Autodesk Inventor part; units mm, degrees
ref_plane "YZ Plane" through (0, 0, 0) normal (1, 0, 0) x (0, 1, 0)
ref_plane "XZ Plane" through (0, 0, 0) normal (0, 1, 0) x (-1, 0, 0)
ref_plane "XY Plane" through (0, 0, 0) normal (0, 0, 1) x (1, 0, 0)
sketch "Sketch1" plane through (0, 0, 0) normal (0, 1, 0) x (-1, 0, 0)
  line L0 (25, 25) -> (-25, 25)
  line L1 (-25, 25) -> (-25, -25)
  line L2 (-25, -25) -> (25, -25)
  line L3 (25, -25) -> (25, 25)
  point P0 (0, 0)
  dimension "d0" = 50
  dimension "d1" = 50
  dimension "d2" = 25
  dimension "d3" = 25
extrude "Extrusion1" add sketch "Sketch1" along normal blind 5
sketch "Sketch2" plane through (0, 0, 0) normal (0, -1, 0) x (1, 0, 0)
  circle A0 centre (0, 0) radius 8
  dimension "d6" = 16
extrude "Extrusion2" add sketch "Sketch2" along normal blind 10
sketch "Sketch3" plane through (0, 5, 0) normal (0, 1, 0) x (1, 0, 0)
  line L0 (0, -3) -> (0, -3)
  line L1 (3, 0) -> (3, 0)
  line L2 (0, 3) -> (0, 3)
  line L3 (-3, 0) -> (-3, 0)
  arc A0 (-3, 0) -> (0, -3) centre (0, 0) ccw
  arc A1 (0, 3) -> (-3, 0) centre (0, 0) ccw
  arc A2 (3, 0) -> (0, 3) centre (0, 0) ccw
  arc A3 (0, -3) -> (3, 0) centre (0, 0) ccw
  point P0 (0, 0)
  dimension "d9" = 6
  dimension "d10" = 6
  dimension "d11" = 3
  dimension "d12" = 3
  dimension "d19" = 3
extrude "Extrusion3" cut sketch "Sketch3" against normal blind 6
sketch "Sketch4" plane through (0, 5, 0) normal (0, 1, 0) x (1, 0, 0)
  line L0 (-5, -5) -> (-5, 5)
  line L1 (-25, 25) -> (-25, -25)
  circle A0 centre (-15, 0) radius 2.5
  line L2 (5, -5) -> (-5, -5)
  line L3 (-5, 5) -> (5, 5)
  circle A1 centre (15, 0) radius 2.5
  line L4 (25, -25) -> (25, 25)
  point P0 (0, 0)
  dimension "d15" = 5
  dimension "d20" = 10
  dimension "d21" = 10
extrude "Extrusion4" cut sketch "Sketch4" against normal blind 3
fillet "Fillet1" radius 5 4 edges at (25, 2.5, 25) (25, 2.5, -25) (-25, 2.5, -25) (-25, 2.5, 25)
sketch "Sketch5" plane through (0, 0, 0) normal (1, 0, 0) x (0, 1, 0)
  line L0 (0, 8) -> (-10, 8)
  line L1 (0, 8) -> (0, 8.5)
  line L2 (0, 20) -> (0, -20)
  line L3 (-10, 8) -> (-10, -8)
  line L4 (-10, 8) -> (0, 8)
  line L5 (-10, 0) -> (0, 0)
  arc A0 (0, 8.5) -> (-10, 8) centre (-2.7668, -36.4149) ccw
  dimension "d23" = 0.5
  dimension "d25" = 45
revolve "Revolution1" add sketch "Sketch5" angle 360 about axis through (0, -10, 0) along (0, 1, 0) contours L0 A0 L1
properties part number "Base"
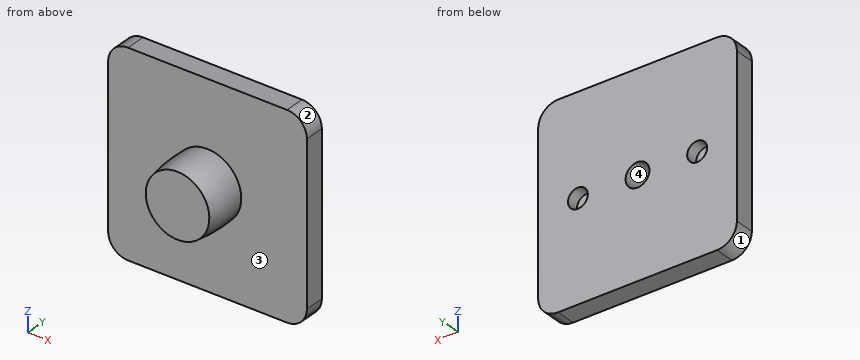
Source: CAD feature listing. Evaluate the final solid. Frame: model axes, mm. Face numbers are marked on the shaded views. Give positions to 0.01 mm unless a question says otherwise; leave off trailing zeros. Write each loop counter-clockwise with the first axis right and the second up, starting at its lowest first coordinate (ties: lowest second). Pieces come first, ordered by that corner, then holes. Notation, with made-up numbers: M 41.25,56.25 L 53.25,56.25 A29 cw 53.25,91.25 Z; hole C 63,72.25 d10. An arc over 180 degrees is marked long. Return JSON: item names as keys, results as strings. Group by question number.
1) Material intervals for line 1 along X through (y, z) = (3.15, 0); line 2 along Z through (x, y) = (-15, 3.95); line 3 along Y through (x, z) = (-14, 4.5), sorted ascending. Write a range as [from, to].
2) Cut plane C-C, the plane z = -15. Output: boundary loops of the cut face in (x, y).
3) Pin query (flat end, axial travel): P1, Ø1.5, axis at x = 14, z = 1, coming from the +Y side; P2, Ø4, axis at x = 7, y = -8, coming from the +Z side; P3, Ø8, axis at x = 7.5, y = -0.5, coming from the -Z side; P4, Ø4, axis at x = -15, z = 0, coming from the -Y side. Return the tip coordinate at first contact, or that it passes through.
4) Cut plane A-A, the plane y = 1. Output: boundary loops of the cut face in (x, z), plus the area to 3 significant figures.
5) Cut plane B-B, the plane x = 15. Output: boundary loops of the cut face in (y, z).
6) Pull-direction query (Z, two-part tool) for the marked faces 1, 2, 3 and 4; classes: pulls with the +Z half, pulls with the -Z half, needs draft (parallel to the pull), parting line crosses it, or undercut.
Recorded:
{
 "1": {"line 1": "x = [-25, -17.5], [-12.5, -3], [3, 12.5], [17.5, 25]", "line 2": "z = [-25, -2.5], [2.5, 25]", "line 3": "y = [0, 5]"},
 "2": {"outline": "M -25,0 L 25,0 L 25,5 L -25,5 Z"},
 "3": {"P1": "stops at y = 2", "P2": "stops at z = 6.63", "P3": "stops at z = -25", "P4": "stops at y = 0"},
 "4": {"outline": "M -25,-20 A5 ccw -20,-25 L 20,-25 A5 ccw 25,-20 L 25,20 A5 ccw 20,25 L -20,25 A5 ccw -25,20 Z; hole C 0,0 d6", "area": "2,450 mm²"},
 "5": {"outline": "M 0,-25 L 5,-25 L 5,-2.5 L 2,-2.5 L 2,2.5 L 5,2.5 L 5,25 L 0,25 Z"},
 "6": {"face 1": "pulls with the -Z half", "face 2": "pulls with the +Z half", "face 3": "needs draft", "face 4": "undercut"}
}
